Design review of the part built by this model. Coordinates are the model's own, in mm. Give positions to 0.01 mm unless a question says otherwise; leave off trailing zeros. Write each loop counter-clockwise with the first axis right and the second up, starting at its lowest first coordinate (ties: lowest second). Pieces come first, ordered by that corner, then holes. Notation, with made-up numbers: M -39.75,46.5 L -5.75,46.5 A5 cw -5.75,53.5 Z; hole C 44.25,71 d8. An arc over 180 degrees is marked long. Write each question's results on one line, items separated by ' | '. Start each with the question number.
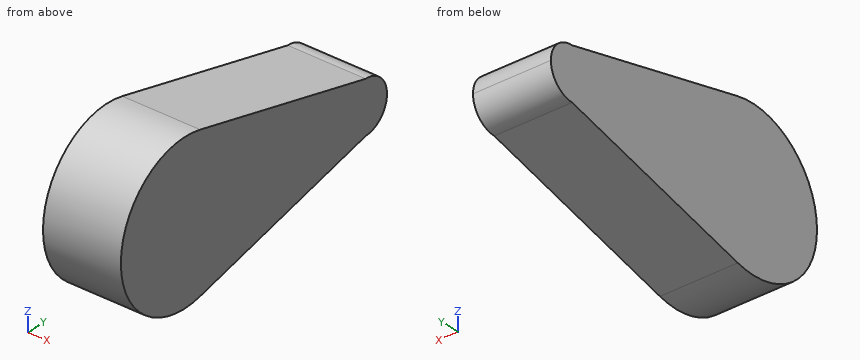
from build123d import *

# Parameters (mm, degrees)
F1_DEPTH = 30


with BuildPart() as f1:
    # F0 (on Right) → F1 (new body)
    with BuildSketch(Plane.YZ):
        with BuildLine():
            ThreePointArc((-37.046180943, -55.3226507139), (-20.6061644078, -44.6968900375), (-14.2198155139, -26.1929585246))
            ThreePointArc((-14.2198155139, -26.1929585246), (-20.6061644078, -7.6890270116), (-37.046180943, 2.9367336647))
            ThreePointArc((-37.046180943, 2.9367336647), (-74.2198155139, -26.1929585246), (-37.046180943, -55.3226507139))
        make_face()
        with BuildLine():
            ThreePointArc((-37.046180943, 2.9367336647), (-20.6061644078, -7.6890270116), (-14.2198155139, -26.1929585246))
            ThreePointArc((-14.2198155139, -26.1929585246), (-20.6061644078, -44.6968900375), (-37.046180943, -55.3226507139))
            Line((-37.046180943, -55.3226507139), (40.6329982284, -36.1929585246))
            ThreePointArc((40.6329982284, -36.1929585246), (30.6329982284, -26.1929585246), (40.6329982284, -16.1929585246))
            Line((40.6329982284, -16.1929585246), (-37.046180943, 2.9367336647))
        make_face()
        with BuildLine():
            ThreePointArc((50.6329982284, -26.1929585246), (47.7040660403, -19.1218907127), (40.6329982284, -16.1929585246))
            ThreePointArc((40.6329982284, -16.1929585246), (30.6329982284, -26.1929585246), (40.6329982284, -36.1929585246))
            ThreePointArc((40.6329982284, -36.1929585246), (47.7040660403, -33.2640263364), (50.6329982284, -26.1929585246))
        make_face()
    extrude(amount=F1_DEPTH)


solid = f1.part
Q1. We need section A-A on x = 22.5. Write out the cut boundary in (y, z).
Q2. We need section B-B on y = 12.5. Write out the cut boundary in (x, z), and give its area (3 significant figures).
Q3. For pin 1 Ø12 at (x, z) = (24.5, -42) entering from -Y; pin 2 Ø12 at (x, y) = (14.5, -53) entering from -Z; pin 3 Ø4 at (x, z) = (22.5, -18.5) entering from -Y, all flat-tipped, find the tip position at first contact; note any pin that passes through.
Q4. Wall thickness on line 1 along Y through (x, z) = (25.5, -26); line 2 along Z through (x, y) = (19.25, -35); line 3 along Z through (x, y) = (27.25, 29): over which ranges is each line inside the solid? List them lowest first. Write a range as from..to.
Q5. We need section C-C on z = -13. Write out the cut boundary in (x, y).
Answer sheet:
1) outline: M -37.05,-55.32 L 40.63,-36.19 A10 ccw 40.63,-16.19 L -37.05,2.94 A30 ccw long Z
2) outline: M 0,-43.12 L 30,-43.12 L 30,-9.26 L 0,-9.26 Z | area: 1,020 mm^2
3) pin 1: y = -72.57 | pin 2: z = -56.06 | pin 3: y = -73.67
4) line 1: -74.22..50.63 | line 2: -54.82..2.43 | line 3: -39.06..-13.33
5) outline: M 0,-71.16 L 30,-71.16 L 30,27.67 L 0,27.67 Z
